from build123d import *

# Parameters (mm, degrees)
F0_W     = 12.7
F0_H     = 25.4
F0_H_2   = 12.7
F1_DEPTH = 2.54
F3_R     = 6.35
F4_DEPTH = 12.7
F5_SIZE  = 6.35
F6_SIZE  = 6.35
F7_R     = 5.08
F8_R     = 3.302


with BuildPart() as f1:
    # F0 (on Front) → F1 (new body)
    with BuildSketch(Plane.XZ):
        with BuildLine():
            Line((38.1, 12.7), (38.1, 25.4))
            Line((38.1, 25.4), (28.398063, 25.4))
            ThreePointArc((28.398063, 25.4), (0, 38.1), (-28.398063, 25.4))
            Line((-28.398063, 25.4), (-38.1, 25.4))
            Line((-38.1, 25.4), (-38.1, 12.7))
            Line((-38.1, 12.7), (-38.1, -12.7))
            Line((-38.1, -12.7), (-38.1, -25.4))
            Line((-38.1, -25.4), (-28.398063, -25.4))
            ThreePointArc((-28.398063, -25.4), (0, -38.1), (28.398063, -25.4))
            Line((28.398063, -25.4), (38.1, -25.4))
            Line((38.1, -25.4), (38.1, -12.7))
            Line((38.1, -12.7), (38.1, 12.7))
        make_face()
        with Locations((44.45, 0)):
            Rectangle(F0_W, F0_H)
        with Locations((-44.45, 19.05)):
            Rectangle(F0_W, F0_H_2)
        with Locations((-44.45, -19.05)):
            Rectangle(F0_W, F0_H_2)
    extrude(amount=F1_DEPTH)

    # F3 (on face) → F4 (cut, symmetric)
    with BuildSketch(Plane.XZ.offset(2.54)):
        Circle(F3_R)
    extrude(amount=F4_DEPTH, both=True, mode=Mode.SUBTRACT)

    # F5
    f5_edges = [f1.edges().sort_by_distance(p)[0] for p in [
        (38.1, -1.27, 25.4),
    ]]
    chamfer(f5_edges, length=F5_SIZE)

    # F6
    f6_edges = [f1.edges().sort_by_distance(p)[0] for p in [
        (38.1, -1.27, -25.4),
    ]]
    chamfer(f6_edges, length=F6_SIZE)

    # F7
    f7_edges = [f1.edges().sort_by_distance(p)[0] for p in [
        (50.8, -1.27, 12.7),
        (50.8, -1.27, -12.7),
    ]]
    fillet(f7_edges, radius=F7_R)

    # F8
    f8_edges = [f1.edges().sort_by_distance(p)[0] for p in [
        (-50.8, -1.27, 25.4),
        (-50.8, -1.27, 12.7),
        (-50.8, -1.27, -25.4),
        (-50.8, -1.27, -12.7),
    ]]
    fillet(f8_edges, radius=F8_R)


solid = f1.part
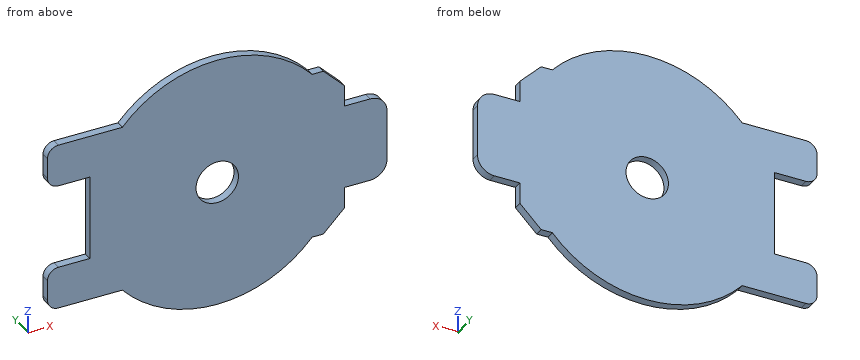
Here's how the part is built. I have some questions about the finished solid (model axes, mm). Round coordinates to 2 decimals unless told otherwise and drop trailing zeros. Loops run counter-clockwise (first coordinate to the right, second up) from the corner with the lowest first, then second, coordinate; pieces in that order, holes last.
1. If I drill on line 1 along Z through (x, y) = (0, -1.4); line 2 along X through (y, z) = (-1.2, 0.5); line 3 along Z through (x, y) = (-32, -0.6), over which ranges is the centre line in solid material (lowest first)?
Answer list:
line 1: z = -38.1 to -6.35, 6.35 to 38.1
line 2: x = -38.1 to -6.33, 6.33 to 50.8
line 3: z = -25.4 to 25.4
2. If we section it at B-B on y = -1.1: Write out the boundary of the cut face in (x, z), plus the area to 3 significant figures.
Answer list:
outline: (-50.8, -22.1) arc R3.3 ccw to (-47.5, -25.4) - (-28.4, -25.4) arc R38.1 ccw to (28.4, -25.4) - (31.75, -25.4) - (38.1, -19.05) - (38.1, -12.7) - (45.72, -12.7) arc R5.08 ccw to (50.8, -7.62) - (50.8, 7.62) arc R5.08 ccw to (45.72, 12.7) - (38.1, 12.7) - (38.1, 19.05) - (31.75, 25.4) - (28.4, 25.4) arc R38.1 ccw to (-28.4, 25.4) - (-47.5, 25.4) arc R3.3 ccw to (-50.8, 22.1) - (-50.8, 16) arc R3.3 ccw to (-47.5, 12.7) - (-38.1, 12.7) - (-38.1, -12.7) - (-47.5, -12.7) arc R3.3 ccw to (-50.8, -16) - close; hole circle Ø12.7 at (0, 0)
area: 5,330 mm2
3. If we section it at C-C on x = 0: Write out the boundary of the cut face in (y, z), plus the area to 3 significant figures.
Answer list:
outline: (-2.54, -38.1) - (0, -38.1) - (0, -6.35) - (-2.54, -6.35) - close; (-2.54, 6.35) - (0, 6.35) - (0, 38.1) - (-2.54, 38.1) - close
area: 161 mm2
4. If we section it at D-D on x = 34.5: Write out the boundary of the cut face in (y, z).
Answer list:
outline: (-2.54, -22.65) - (0, -22.65) - (0, 22.65) - (-2.54, 22.65) - close
5. If we section it at A-A on z = 0: Write out the boundary of the cut face in (x, y).
Answer list:
outline: (-38.1, -2.54) - (-6.35, -2.54) - (-6.35, 0) - (-38.1, 0) - close; (6.35, -2.54) - (50.8, -2.54) - (50.8, 0) - (6.35, 0) - close
6. For P1, Ø1.3, axis at x = -45, y = -1, coming from the -Z side; P2, Ø7.5, axis at x = 0, z = 0, coming from the +Y side; P3, Ø1, axis at y = -2, z = 25.5, coming from the -X side; P4, Ø5, axis at x = 0, z = -21.5, coming from the +Y side, each with a flat end and sliding along its axis, tell me the tip position at first contact or that it passes through.
Answer list:
P1: stops at z = -25.4
P2: passes through
P3: stops at x = -49.07
P4: stops at y = 0
